Design review of the part built by this model. Coordinates are the model's own, in mm. Face numbers are marked on the shaded views. A direction names the side the tool comes from. Round coordinates to 2 decimals unless told otherwise and drop trailing zeros. Loops run counter-clockwise (first coordinate to the right, second up) from the corner with the lowest first, then second, coordinate; pieces in that order, holes last. Notation, with made-up numbers: M 40.5,58.25 L 48.5,58.25 A29 cw 48.5,90.25 Z; hole C 28.25,13 d7. An arc over 180 degrees is marked long. One line per item, written item: value. Start each with the question number.
Item 1: For line 1 along Y through (x, z) = (-0.7, 0); line 2 along Z through (x, y) = (-1.75, -22); line 3 along X through (y, z) = (-30.5, -5), list the stretches that pass through material, from the lowest coordinate up.
Item 2: Clearance check with flat-ended pins moving along their axes: pin 1 (5 mm diameter, centred on y = -21.8, z = 12.54, fed in from -X); pin 2 (5 mm diameter, centred on x = -19.5, y = 0, fed in from +Z); pin 3 (6 mm diameter, centred on x = -5.5, z = 24, fed in from -Y). State where each tip first meets the part, or that it passes through.
Item 3: We need section C-C (x = -13.25). Write out the cut boundary in (y, z), then the cut area to 3 significant figures.
Item 4: We need section D-D (y = -15.5). Write out the cut boundary in (x, z).
Item 5: We need section A-A (z = 0). Write out the cut boundary in (x, y).
Item 6: We need section B-B (x = -19.5). Write out the cut boundary in (y, z).
Item 7: For the marked faces 3 and 4, list the 3-axis set-ups (+Z, -Z, +X, -X, +Y, -Y) from which the entire face can be reached by the end or side of a thin tool; tool diameter is ignored.
Item 8: Mouldability with a two-part tool opening along Y and no side actions: class the marked faces 1 and 2 as released by +Y, released by -Y, zero draft, split by the parting line, or undercut.
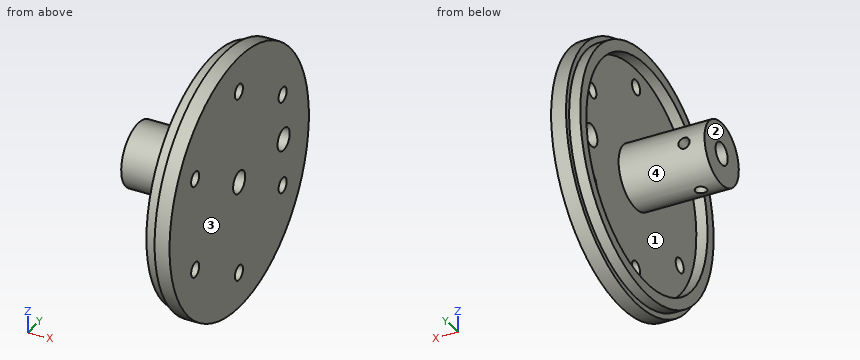
from build123d import *

# Parameters (mm, degrees)
SKETCH1_R           = 34.5
BOSS_EXTRUDE1_DEPTH = 2
SKETCH2_R           = 8.49
BOSS_EXTRUDE2_DEPTH = 23
SKETCH4_R           = 3
CUT_EXTRUDE1_DEPTH  = 30
CUT_EXTRUDE2_REACH  = 45
SKETCH5_R           = 1.5
CUT_EXTRUDE3_REACH  = 36.5
SKETCH6_R           = 1.5
SKETCH19_R          = 33
SKETCH19_R_2        = 30
BOSS_EXTRUDE5_DEPTH = 3
SKETCH21_R          = 3
CUT_EXTRUDE6_DEPTH  = 10
SKETCH20_R          = 2
CUT_EXTRUDE7_DEPTH  = 10


with BuildPart() as part:
    # Sketch1 → Boss-Extrude1 (new body, symmetric)
    with BuildSketch(Plane(origin=(0, 0, 0), x_dir=(0, 0, -1), z_dir=(1, 0, 0))):
        Circle(SKETCH1_R)
    extrude(amount=BOSS_EXTRUDE1_DEPTH, both=True)

    # Sketch2 → Boss-Extrude2 (add)
    with BuildSketch(Plane.ZY.offset(2)):
        Circle(SKETCH2_R)
    extrude(amount=BOSS_EXTRUDE2_DEPTH)

    # Sketch4 → Cut-Extrude1 (cut)
    with BuildSketch(Plane.ZY.offset(25)):
        Circle(SKETCH4_R)
    extrude(amount=-CUT_EXTRUDE1_DEPTH, mode=Mode.SUBTRACT)

    # Sketch5 → Cut-Extrude2 (cut, up to next)
    with BuildSketch(Plane(origin=(0, 8.5, 0), x_dir=(1, 0, 0), z_dir=(0, 1, 0)), mode=Mode.PRIVATE) as cut_extrude2_sk1:
        with Locations((-19.5, 0)):
            Circle(SKETCH5_R)
    cut_extrude2_tool1 = extrude(cut_extrude2_sk1.sketch, amount=-CUT_EXTRUDE2_REACH, mode=Mode.PRIVATE) & part.part
    add(cut_extrude2_tool1.solids().sort_by_distance((-19.5, 8.5, 0))[0], mode=Mode.SUBTRACT)

    # Sketch6 → Cut-Extrude3 (cut, up to next)
    with BuildSketch(Plane.XY, mode=Mode.PRIVATE) as cut_extrude3_sk1:
        with Locations((-19.5, 0)):
            Circle(SKETCH6_R)
    cut_extrude3_tool1 = extrude(cut_extrude3_sk1.sketch, amount=-CUT_EXTRUDE3_REACH, mode=Mode.PRIVATE) & part.part
    add(cut_extrude3_tool1.solids().sort_by_distance((-19.5, 0, 0))[0], mode=Mode.SUBTRACT)

    # Sketch19 → Boss-Extrude5 (add)
    with BuildSketch(Plane.ZY.offset(2)):
        Circle(SKETCH19_R)
        Circle(SKETCH19_R_2, mode=Mode.SUBTRACT)
    extrude(amount=BOSS_EXTRUDE5_DEPTH)

    # Sketch21 → Cut-Extrude6 (cut)
    with BuildSketch(Plane.ZY.offset(2)):
        with Locations((0, 22)):
            Circle(SKETCH21_R)
    extrude(amount=-CUT_EXTRUDE6_DEPTH, mode=Mode.SUBTRACT)

    # Sketch20 → Cut-Extrude7 (cut)
    with BuildSketch(Plane.ZY.offset(2)):
        with Locations((-12.422389037, 21.516208963)):
            Circle(SKETCH20_R)
        with Locations((12.577603677, 21.497122149)):
            Circle(SKETCH20_R)
        with Locations((25.061070367, -0.163050043)):
            Circle(SKETCH20_R)
        with Locations((12.544544344, -21.804135421)):
            Circle(SKETCH20_R)
        with Locations((-12.45544837, -21.785048606)):
            Circle(SKETCH20_R)
        with Locations((-24.93891506, -0.124876414)):
            Circle(SKETCH20_R)
    extrude(amount=-CUT_EXTRUDE7_DEPTH, mode=Mode.SUBTRACT)


solid = part.part
A:
1. line 1: -34.5 to -3, 3 to 19, 25 to 34.5
1. line 2: -26.58 to -14.44, -10.47 to 10.55, 14.53 to 26.58
1. line 3: -5 to 2
2. pin 1: x = -2
2. pin 2: z = 8.49
2. pin 3: y = -25.42
3. outline: C 0,0 d16.98; hole C 0,0 d6
3. area: 198 mm2
4. outline: M -5,-29.13 L -2,-29.13 L -2,-30.82 L 2,-30.82 L 2,30.82 L -2,30.82 L -2,29.13 L -5,29.13 L -5,25.69 L -2,25.69 L -2,-25.69 L -5,-25.69 Z
5. outline: M -25,-8.49 L -2,-8.49 L -2,-30 L -5,-30 L -5,-33 L -2,-33 L -2,-34.5 L 2,-34.5 L 2,-3 L -25,-3 Z; M -25,3 L -21,3 L -21,8.49 L -25,8.49 Z; M -18,3 L 2,3 L 2,19 L -2,19 L -2,8.49 L -18,8.49 Z; M -5,30 L -2,30 L -2,25 L 2,25 L 2,34.5 L -2,34.5 L -2,33 L -5,33 Z
6. outline: M -1.5,-8.36 L -1.5,-2.6 A3 cw long 2.6,1.5 L 8.36,1.5 A8.49 ccw long Z; M 1.5,-8.36 A8.49 ccw 8.36,-1.5 L 2.6,-1.5 A3 cw 1.5,-2.6 Z
7. face 3: +Z, -Z, +X, +Y, -Y
7. face 4: -X
8. face 1: undercut
8. face 2: zero draft
